The model under review builds one solid part; all positions refer to its coordinate system, in mm. Face numbers are marked on the shaded views. Round coordinates to 2 decimals unless told otherwise and drop trailing zeros. Loops run counter-clockwise (first coordinate to the right, second up) from the corner with the lowest first, then second, coordinate; pieces in that order, holes last. Notation, with made-up numbers: M -18,69 L 20,69 A24 ccw 20,79 Z; hole C -32,75.25 d1. An arc over 180 degrees is marked long. Answer in a Markdown table with one row per item. Add a question column.
from build123d import *

# Parameters (mm, degrees)
F2_SIZE = 1


# Not quite as in the source:
# - a fillet or chamfer that OpenCascade refuses, or shapes differently, is made with other operations: its cross-section is extruded or revolved along the edge and cut away or added


with BuildPart() as f1:
    # F0 (on Front) → F1 (revolve)
    with BuildSketch(Plane.XZ):
        with BuildLine():
            Line((-5.2, 0), (-5.2, 20.18))
            Line((-5.2, 20.18), (-14, 20.18))
            ThreePointArc((-14, 20.18), (-12, 10.09), (-14, 0))
            Line((-14, 0), (-5.2, 0))
        make_face()
    revolve(axis=Axis((0, 0, 10.09), (0, 0, 1)))

    # F2
    f2_edges = [f1.edges().sort_by_distance(p)[0] for p in [
        (5.2, 0, 0),
        (5.2, 0, 20.18),
        (-5.2, 0, 10.09),
    ]]
    chamfer(f2_edges, length=F2_SIZE)

    # F3: chamfer of 2 on 3 edges, made by hand

    # F3_s1 → F3_t2 (revolve, cut)
    with BuildSketch(Plane.XZ):
        with BuildLine():
            Line((-13.3927401151, 18.3553817289), (-12.0288953822, 20.2448671044))
            Line((-12.0288953822, 20.2448671044), (-12.0288953822, 20.2848671044))
            ThreePointArc((-12.0288953822, 20.2848671044), (-13.0144476911, 20.22), (-14, 20.22))
            Line((-14, 20.22), (-14.0369756569, 20.1647421889))
            ThreePointArc((-14.0369756569, 20.1647421889), (-13.6870919943, 19.2711305309), (-13.4307048554, 18.3427849635))
            Line((-13.4307048554, 18.3427849635), (-13.3927401151, 18.3553817289))
        make_face()
    revolve(axis=Axis((0, 0, 20.18), (0, 0, 1)), mode=Mode.SUBTRACT)

    # F3_s3 → F3_t4 (revolve, cut)
    with BuildSketch(Plane.XZ):
        with BuildLine():
            Line((-12.0288953822, -0.0648671044), (-13.3927401151, 1.8246182711))
            Line((-13.3927401151, 1.8246182711), (-13.4307048554, 1.8372150365))
            ThreePointArc((-13.4307048554, 1.8372150365), (-13.6870919943, 0.9088694691), (-14.0369756569, 0.0152578111))
            Line((-14.0369756569, 0.0152578111), (-14, -0.04))
            ThreePointArc((-14, -0.04), (-13.0144476911, -0.04), (-12.0288953822, -0.1048671044))
            Line((-12.0288953822, -0.1048671044), (-12.0288953822, -0.0648671044))
        make_face()
    revolve(axis=Axis((0, 0, 0), (0, 0, 1)), mode=Mode.SUBTRACT)


solid = f1.part
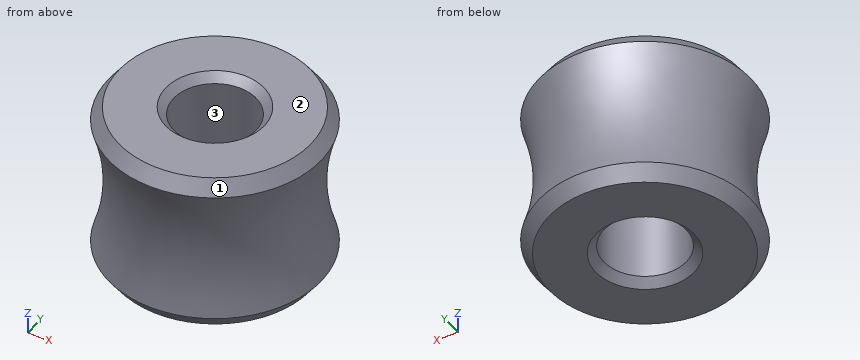
1. Take a section at C-C, the plane z = 10.5. State the section outline as (x, y) points, and give its area (3 significant figures).
2. Take a section at D-D, the plane z = 16.75. State the section outline as (x, y) points, and give its area (3 significant figures).
3. To check wall thickness, follow probe 1 along Y at (x, z) = (0, 14.75); probe 2 along Y at (x, z) = (-2, 8); probe 3 along X at (y, z) = (-0.75, 7.25). State the ranges of each line that lie inside material, in increasing order.
4. Take a section at A-A, the plane x = 0. State the section outline as (y, z) points, and give its area (3 significant figures).
5. For pin 1 Ø1.5 at (x, z) = (9, 2.5) entering from +Y; pin 2 Ø6 at (x, z) = (5.5, 2) entering from +Y; pin 3 Ø8 at (x, z) = (10.5, 16) entering from -Y; pin 4 Ø6 at (x, y) = (-1, 8) entering from -Z, all flat-tipped, find the tip position at first contact; note any pin that passes through.
6. Mouldability with a two-part tool opening along X and no side actions: class the marked faces 1, 2 and 3 as released by +X, released by -X, zero draft, split by the parting line, or undercut.
Check sheet entries:
| question | item | result |
|---|---|---|
| 1 | outline | C 0,0 d24.01; hole C 0,0 d10.4 |
| 1 | area | 368 mm^2 |
| 2 | outline | C 0,0 d25.7; hole C 0,0 d10.4 |
| 2 | area | 434 mm^2 |
| 3 | probe 1 | y = -12.41 to -5.2, 5.2 to 12.41 |
| 3 | probe 2 | y = -11.92 to -4.8, 4.8 to 11.92 |
| 3 | probe 3 | x = -12.13 to -5.15, 5.15 to 12.13 |
| 4 | outline | M -13.35,1.76 L -12.08,0 L -6.2,0 L -5.2,1 L -5.2,19.18 L -6.2,20.18 L -12.08,20.18 L -13.35,18.42 A26.45 cw Z; M 5.2,1 L 6.2,0 L 12.08,0 L 13.35,1.76 A26.45 cw 13.35,18.42 L 12.08,20.18 L 6.2,20.18 L 5.2,19.18 Z |
| 4 | area | 292 mm^2 |
| 5 | pin 1 | stops at y = 10.26 |
| 5 | pin 2 | stops at y = 13.11 |
| 5 | pin 3 | stops at y = -11.18 |
| 5 | pin 4 | stops at z = 0 |
| 6 | face 1 | split by the parting line |
| 6 | face 2 | zero draft |
| 6 | face 3 | undercut |
